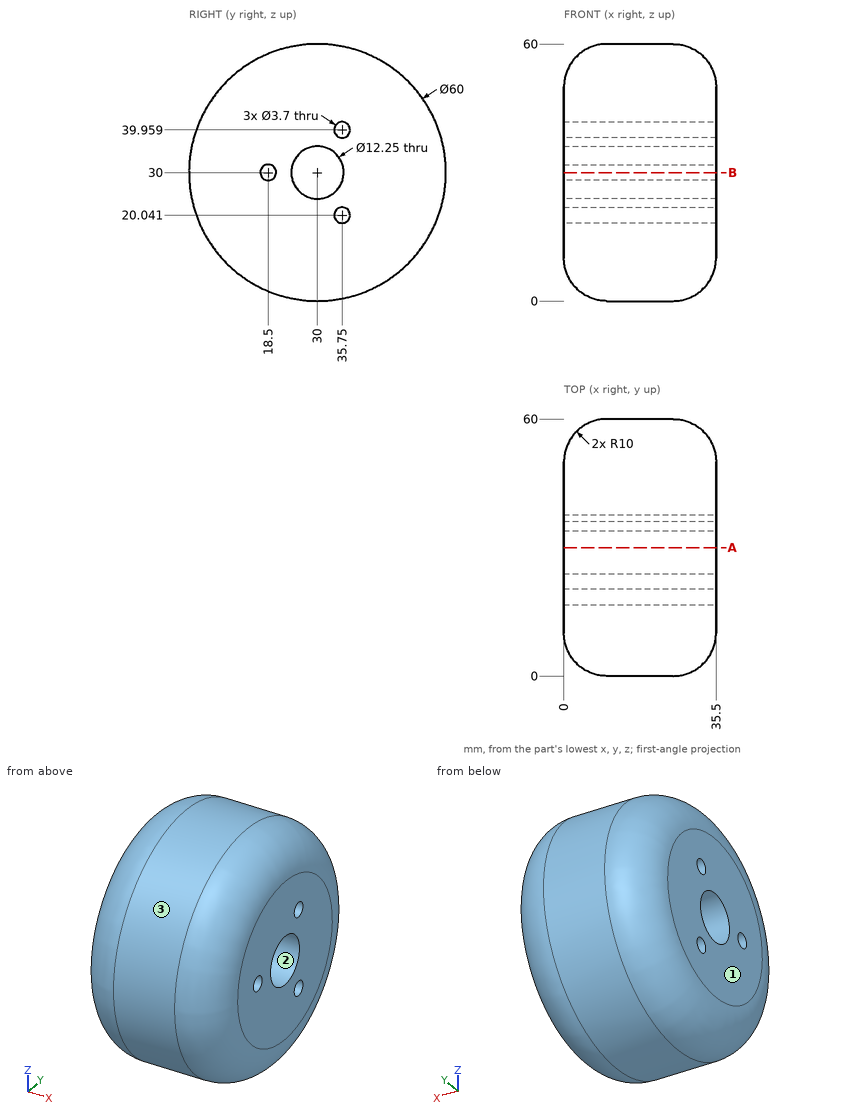
Geometry check sheet. Reference: drawing and pictorial views, mm from the part's lowest x, y, z. Give positions to 0.01 mm unless a question says otherwise; leave off trailing zeros. Write each loop counter-clockwise with the first axis right and the second up, starting at its lowest first coordinate (ties: lowest second). Pieces come first, ordered by that corner, then holes. Notation, with made-up numbers: (26, -11.5) - (48, -11.5) arc R10 cw to (48, -7.5) - close; hole circle Ø3 at (-11.75, 74). An arc over 180 degrees is marked (long way). Put each result on its own line as item: value.
Q1. Scan lines: probe 1 along Z at (x, y) = (15, 35); probe 2 along Z at (x, y) = (24.5, 35.5) (1 decimal); probe 3 along Y at (x, z) = (25, 40) (1 decimal). Record each from-to range of solid material in increasing order. Write a range as from..to.
Result:
probe 1: 0.42..18.35, 21.73..26.46, 33.54..38.27, 41.65..59.58
probe 2: 0.5..18.2, 21.9..27.3, 32.7..38.1, 41.8..59.5
probe 3: 1.7..33.9, 37.6..58.3
Q2. Section check B-B on z = 30. Count the separate pieces of the cut face and the enclosed holes in it, and give its area (3 significant figures).
Result:
separate pieces: 3
enclosed holes: 0
area: 1,480 mm2
Q3. Mould release check, pull along Y, two halves, no side actions. Record for the marked faces 1, 2 and 3: released by +Y, released by -Y, zero draft, split by the parting line, or undercut.
Result:
face 1: zero draft
face 2: undercut
face 3: split by the parting line
Q4. Depth check by flat-ended pin: P1, Ø6, axis at x = 8, y = 33, coming from the -Z side; P2, Ø10, axis at x = 15, y = 17.5, coming from the +Z side; P3, Ø1, axis at x = 30, y = 14, coming from the -Z side. Enter the tip coordinate at first touch or a pass-through.
Result:
P1: z = 0.01
P2: z = 59.05
P3: z = 5.46
Q5. Section check A-A on y = 30. Record the cut outline in (x, z) (1 decimal).
Result:
outline: (0, 10) arc R10 ccw to (10, 0) - (25.5, 0) arc R10 ccw to (35.5, 10) - (35.5, 23.9) - (0, 23.9) - close; (0, 36.1) - (35.5, 36.1) - (35.5, 50) arc R10 ccw to (25.5, 60) - (10, 60) arc R10 ccw to (0, 50) - close
